Verification items for the finished model (mm, model axes). A direction names the side the tool comes from. Coordinates: 2 decimals unless noted, no trailing zeros. Order: outer loops, then holes, each group sorted by start corner. A loop starts at its lowest first (then second) coordinate and runs counter-clockwise, first axis right, second up.
Q1. Cross-section at C-C, the plane x = -13.5. Record the boundary of the cut face in (y, z).
Q2. Draft check along X on faces 3 (the flat face through (5, 0, 54)), 4 (the cylindrical face through (36.264, -5.81, 58.21)), 5 (the flat face through (-3, 1.5, 45)). Enter one of: pulls with the +X half, pulls with the -X half, needs draft (parallel to the pull), parting line crosses it, or undercut.
Q3. Set-up check for faces 1 (the cylindrical face through (-13.06, -4.93, 48.68)), 2 (the cylindrical face through (-4.21, 0.6, 31.77)): record each of +Z, -Z, +X, -X, +Y, -Y from which the full face is reachable in a straight line by a thin tool's end or side.
Q4. Thickness scan on line 1 (Z direction, x = 2, y = -3); line 2 (Z direction, x = 7.5, y = -3.75); line 3 (Y direction, x = -14, z = 36.75). Record the ranges inside material, lowest first.
Q5. Depth check by flat-ended pin: P1, Ø6, axis at x = 31.92, z = 53.91, coming from the -Y side. Enter the tip coordinate at first touch or a pass-through.
Q6. Cross-section at B-B, the plane y = -5. Count the separate pieces of the cut face and the enclosed holes in it, and give its area (3 significant figures).
Q7. Cross-section at A-A, the plane x = -37.5. Record the boundary of the cut face in (y, z).
Q8. Cross-section at D-D, the plane y = 0.75. Record the boundary of the cut face in (x, z).
from build123d import *

# Parameters (mm, degrees)
F0_W     = 81.6
F0_H     = 28.2
F0_R     = 3.7
F1_DEPTH = 10
F2_W     = 81.6
F2_H     = 28.2
F3_DEPTH = 1.5
F4_R     = 3


with BuildPart() as f1:
    # F0 (on Front) → F1 (new body)
    with BuildSketch(Plane.XZ):
        with Locations((-3.680077, 45.012411)):
            Rectangle(F0_W, F0_H)
        with Locations((-39.280077, 36.112411)):
            Circle(F0_R, mode=Mode.SUBTRACT)
        with Locations((-30.380077, 36.112411)):
            Circle(F0_R, mode=Mode.SUBTRACT)
        with Locations((-21.480077, 36.112411)):
            Circle(F0_R, mode=Mode.SUBTRACT)
        with Locations((-12.580077, 36.112411)):
            Circle(F0_R, mode=Mode.SUBTRACT)
        with Locations((-3.680077, 36.112411)):
            Circle(F0_R, mode=Mode.SUBTRACT)
        with Locations((5.219923, 36.112411)):
            Circle(F0_R, mode=Mode.SUBTRACT)
        with Locations((14.119923, 36.112411)):
            Circle(F0_R, mode=Mode.SUBTRACT)
        with Locations((23.019923, 36.112411)):
            Circle(F0_R, mode=Mode.SUBTRACT)
        with Locations((31.919923, 36.112411)):
            Circle(F0_R, mode=Mode.SUBTRACT)
        with Locations((-39.280077, 45.012411)):
            Circle(F0_R, mode=Mode.SUBTRACT)
        with Locations((-30.380077, 45.012411)):
            Circle(F0_R, mode=Mode.SUBTRACT)
        with Locations((-21.480077, 45.012411)):
            Circle(F0_R, mode=Mode.SUBTRACT)
        with Locations((-12.580077, 45.012411)):
            Circle(F0_R, mode=Mode.SUBTRACT)
        with Locations((-39.280077, 53.912411)):
            Circle(F0_R, mode=Mode.SUBTRACT)
        with Locations((-30.380077, 53.912411)):
            Circle(F0_R, mode=Mode.SUBTRACT)
        with Locations((-21.480077, 53.912411)):
            Circle(F0_R, mode=Mode.SUBTRACT)
        with Locations((-12.580077, 53.912411)):
            Circle(F0_R, mode=Mode.SUBTRACT)
        with Locations((-3.680077, 45.012411)):
            Circle(F0_R, mode=Mode.SUBTRACT)
        with Locations((5.219923, 45.012411)):
            Circle(F0_R, mode=Mode.SUBTRACT)
        with Locations((14.119923, 45.012411)):
            Circle(F0_R, mode=Mode.SUBTRACT)
        with Locations((23.019923, 45.012411)):
            Circle(F0_R, mode=Mode.SUBTRACT)
        with Locations((31.919923, 45.012411)):
            Circle(F0_R, mode=Mode.SUBTRACT)
        with Locations((-3.680077, 53.912411)):
            Circle(F0_R, mode=Mode.SUBTRACT)
        with Locations((5.219923, 53.912411)):
            Circle(F0_R, mode=Mode.SUBTRACT)
        with Locations((14.119923, 53.912411)):
            Circle(F0_R, mode=Mode.SUBTRACT)
        with Locations((23.019923, 53.912411)):
            Circle(F0_R, mode=Mode.SUBTRACT)
        with Locations((31.919923, 53.912411)):
            Circle(F0_R, mode=Mode.SUBTRACT)
        with Locations((31.919923, 45.012411)):
            Circle(F0_R)
    extrude(amount=F1_DEPTH)

    # F2 (on face) → F3 (join)
    with BuildSketch(Plane(origin=(0, 0, 0), x_dir=(-1, 0, 0), z_dir=(0, 1, 0))):
        with Locations((3.680077, 45.012411)):
            Rectangle(F2_W, F2_H)
    extrude(amount=F3_DEPTH)

    # F4
    f4_edges = [f1.edges().sort_by_distance(p)[0] for p in [
        (-44.480077, -4.25, 30.912411),
        (-44.480077, -4.25, 59.112411),
        (37.119923, -4.25, 30.912411),
        (37.119923, -4.25, 59.112411),
        (-3.680077, 1.5, 59.112411),
        (37.119923, 1.5, 45.012411),
        (-3.680077, 1.5, 30.912411),
        (-44.480077, 1.5, 45.012411),
    ]]
    fillet(f4_edges, radius=F4_R)


solid = f1.part
Check values:
1. outline: (-10, 30.91) - (-1.5, 30.91) arc R3 ccw to (1.5, 33.91) - (1.5, 56.11) arc R3 ccw to (-1.5, 59.11) - (-10, 59.11) - (-10, 57.5) - (0, 57.5) - (0, 50.33) - (-10, 50.33) - (-10, 48.6) - (0, 48.6) - (0, 41.43) - (-10, 41.43) - (-10, 39.7) - (0, 39.7) - (0, 32.53) - (-10, 32.53) - close
2. face 3: undercut
2. face 4: pulls with the +X half
2. face 5: needs draft
3. face 1: -Y
3. face 2: -Z, +X, -X, +Y
4. line 1: z = 30.91 to 34.29, 37.94 to 43.19, 46.84 to 52.09, 55.74 to 59.11
4. line 2: z = 30.91 to 33.2, 39.03 to 42.1, 47.93 to 51, 56.83 to 59.11
4. line 3: y = 0 to 1.5
5. P1: stops at y = 0
6. separate pieces: 1
6. enclosed holes: 26
6. area: 1,180 mm2
7. outline: (-10, 30.91) - (-1.5, 30.91) arc R3 ccw to (1.5, 33.91) - (1.5, 56.11) arc R3 ccw to (-1.5, 59.11) - (-10, 59.11) - (-10, 57.16) - (0, 57.16) - (0, 50.67) - (-10, 50.67) - (-10, 48.26) - (0, 48.26) - (0, 41.77) - (-10, 41.77) - (-10, 39.36) - (0, 39.36) - (0, 32.87) - (-10, 32.87) - close
8. outline: (-43.46, 33.91) arc R1.98 ccw to (-41.48, 31.93) - (34.12, 31.93) arc R1.98 ccw to (36.1, 33.91) - (36.1, 56.11) arc R1.98 ccw to (34.12, 58.1) - (-41.48, 58.1) arc R1.98 ccw to (-43.46, 56.11) - close
